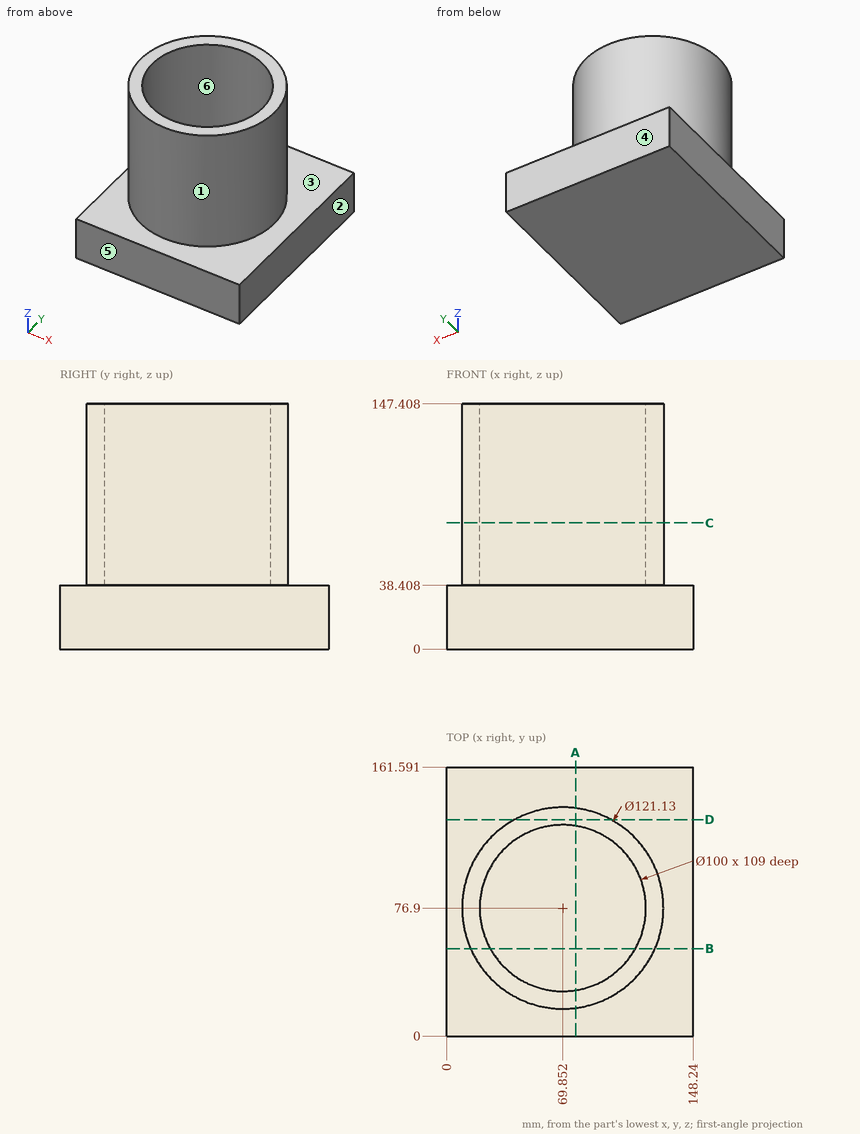
Part print with two shaded views. Sizes in mm from the minimum x, y, z corner. A direction names the side the tool comes from. Round coordinates to 2 decimals unless told otherwise and drop trailing zeros. Write each loop counter-clockwise with the first axis right and the second up, starting at its lowest first coordinate (ties: lowest second). Pieces come first, ordered by that corner, then holes. Notation, with made-up numbers: (-0.75, -15.75) - (30.25, -15.75) arc R18 ccw to (30.25, -6.75) - close; hole circle Ø11 at (36.5, -37). An arc over 180 degrees is marked (long way). Use CSV: the item, a comma, the result in double quotes.
Item 1: Slice it at A-A, the plane x = 77.5. Write the cut outline in (y, z), then the cut area to 3 significant figures.
Results list:
outline,"(0, 0) - (161.59, 0) - (161.59, 38.41) - (136.98, 38.41) - (136.98, 147.41) - (126.31, 147.41) - (126.31, 38.41) - (27.49, 38.41) - (27.49, 147.41) - (16.82, 147.41) - (16.82, 38.41) - (0, 38.41) - close"
area,"8,530 mm²"
Item 2: Pull direction Y, two halves, no side cores. Call the marked faces 3, 4, 5 and 6: pulls with the +Y half, pulls with the -Y half, needs draft (parallel to the pull), parting line crosses it, or undercut.
Results list:
face 3,"needs draft"
face 4,"pulls with the +Y half"
face 5,"pulls with the -Y half"
face 6,"undercut"
Item 3: Wall check: L1, parallel to Z at x = 14, y = 20; L2, parallel to X at y = 119.5, z = 111.5 (1 decimal); L3, parallel to Y at x = 50.5, z = 61. Give the ranges that are in metal, low to high.
Results list:
L1,"z = 0 to 38.41"
L2,"x = 26.8 to 43.7, 96 to 112.9"
L3,"y = 19.51 to 30.8, 123 to 134.29"
Item 4: Slice it at C-C, the plane z = 76. Write the cut outline in (x, y) (1 decimal), then the cut area to 3 significant figures.
Results list:
outline,"circle Ø121.1 at (69.9, 76.9); hole circle Ø100 at (69.9, 76.9)"
area,"3,670 mm²"
Item 5: Tool access for the marked faces 1 and 2: list every direction of +Z, -Z, +X, -X, +Y, -Y with a clear straight run to the whole face (end or side of a thin tool).
Results list:
face 1,"+Z"
face 2,"+Z, -Z, +X, +Y, -Y"
Item 6: Slice it at B-B, the plane y = 52.5. Write the cut outline in (x, z) (1 decimal).
Results list:
outline,"(0, 0) - (148.2, 0) - (148.2, 38.4) - (125.3, 38.4) - (125.3, 147.4) - (113.5, 147.4) - (113.5, 38.4) - (26.2, 38.4) - (26.2, 147.4) - (14.4, 147.4) - (14.4, 38.4) - (0, 38.4) - close"
Item 7: Slice it at D-D, the plane y = 130. Write the cut outline in (x, z).
Results list:
outline,"(0, 0) - (148.24, 0) - (148.24, 38.41) - (98.98, 38.41) - (98.98, 147.41) - (40.72, 147.41) - (40.72, 38.41) - (0, 38.41) - close"
Item 8: Flat gauge pins, fed straight in: P1, Ø1.5, axis at y = 36, z = 126, coming from the +X side; P2, Ø3, axis at x = 31, z = 90.5, coming from the +Y side (1 decimal); P3, Ø10, axis at x = 27, z = 90.5, coming from the -Y side. Where does each tip first touch, or does it go through?
Results list:
P1,"stops at x = 115.2"
P2,"stops at y = 124.6"
P3,"stops at y = 29.62"
